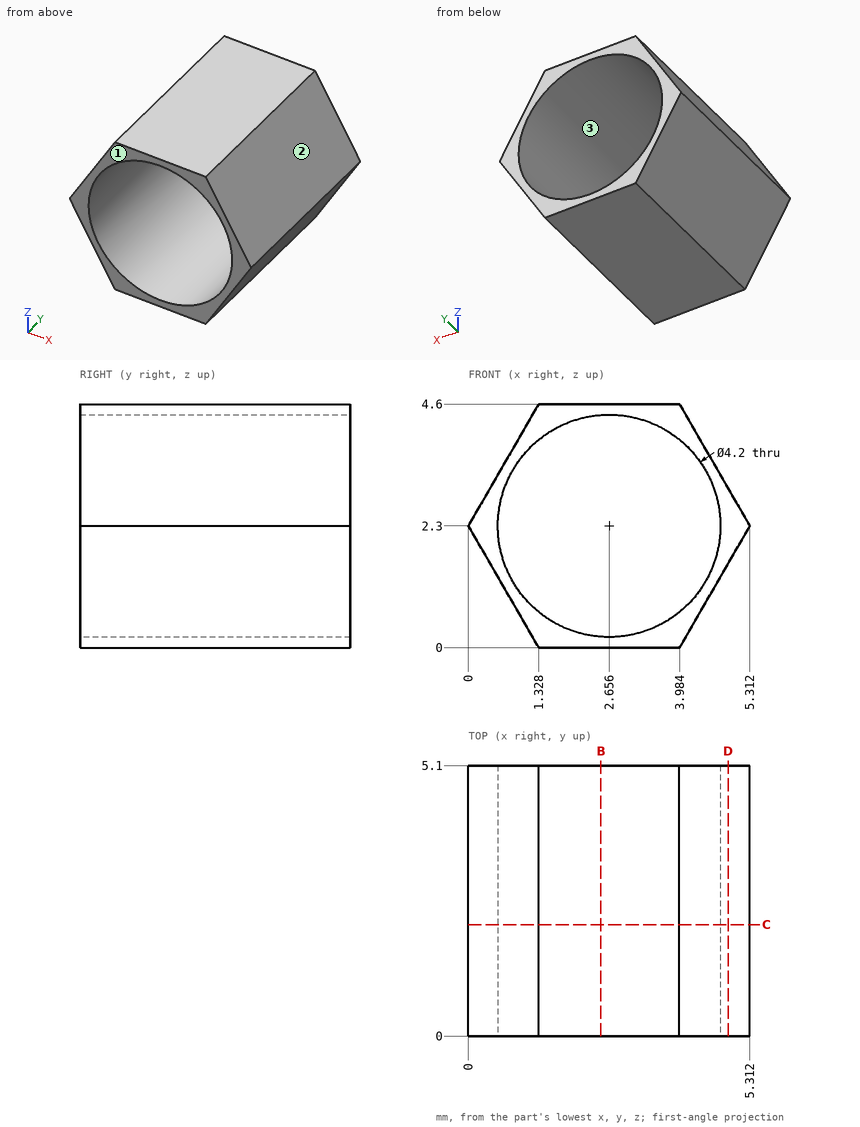
Source: three-view drawing plus pictorial views. Frame: mm from the lowest corner of the part. Give positions to 0.01 mm unless a question says otherwise; leave off trailing zeros. Write each loop counter-clockwise with the first axis right and the second up, starting at its lowest first coordinate (ties: lowest second). Pieces come first, ordered by that corner, then holes. Notation, with made-up numbers: (68.25, 66.5) - (103.25, 66.5) arc R24 cw to (103.25, 76.5) - close; hole circle Ø6 at (-34, 20). An arc over 180 degrees is marked (long way). Write item = value, one per line. Start each with the question number.
Q1. Cut plane C-C, the plane y = 2.1. Return loops of the section in (x, z).
Q2. Cut plane D-D, the plane x = 4.9. Return loops of the section in (y, z).
Q3. Pin query (flat end, axial travel): pin 1 Ø1 at (y, z) = (4, 3) entering from +X. Return the tip coordinate at first contact, or that it passes through.
Q4. Material intervals for probe 1 along X at (y, z) = (0.85, 3.5); probe 2 along Z at (x, y) = (3.9, 4.4); probe 3 along X at (y, z) = (4.75, 2.5) (1 decimal), sorted ascending.
Q5. Draft query along X for the marked faces 1, 2 and 3. Return one class per face: +X half, -X half, draft (parallel to the pull), parting line (faces both ways), or undercut.
Q6. Cut plane B-B, the plane x = 2.5. Return loops of the section in (y, z).
Computed values:
q1.outline = (0, 2.3) - (1.33, 0) - (3.98, 0) - (5.31, 2.3) - (3.98, 4.6) - (1.33, 4.6) - close; hole circle Ø4.2 at (2.66, 2.3)
q2.outline = (0, 1.59) - (5.1, 1.59) - (5.1, 3.01) - (0, 3.01) - close
q3.pin_1 = 5.2
q4.probe_1 = 0.69 to 0.93, 4.38 to 4.62
q4.probe_2 = 0 to 0.61, 3.99 to 4.6
q4.probe_3 = 0.1 to 0.6, 4.7 to 5.2
q5.face_1 = draft
q5.face_2 = +X half
q5.face_3 = undercut
q6.outline = (0, 0) - (5.1, 0) - (5.1, 0.21) - (0, 0.21) - close; (0, 4.39) - (5.1, 4.39) - (5.1, 4.6) - (0, 4.6) - close
